from build123d import *

# Parameters (mm, degrees)
SKETCH1_W           = 35
SKETCH1_H           = 45
BOSS_EXTRUDE1_DEPTH = 6
SKETCH2_W           = 45
SKETCH2_H           = 17
BOSS_EXTRUDE2_DEPTH = 5
SKETCH3_R           = 1
CUT_EXTRUDE1_DEPTH  = 5
SKETCH3_2_R         = 1
CUT_EXTRUDE2_DEPTH  = 30
SKETCH4_R           = 2
CUT_EXTRUDE3_DEPTH  = 5
FILLET1_R           = 0.762
FILLET2_R           = 10
FILLET3_R           = 1
CUT_EXTRUDE4_DEPTH  = 23
SKETCH6_R           = 1.5
CUT_EXTRUDE5_DEPTH  = 6


with BuildPart() as part:
    # Sketch1 → Boss-Extrude1 (new body)
    with BuildSketch(Plane(origin=(0, 0, 0), x_dir=(1, 0, 0), z_dir=(0, 1, 0))):
        Rectangle(SKETCH1_W, SKETCH1_H)
    extrude(amount=BOSS_EXTRUDE1_DEPTH)

    # Sketch2 → Boss-Extrude2 (add)
    with BuildSketch(Plane.ZY.offset(17.5)):
        with Locations((0, 14.5)):
            Rectangle(SKETCH2_W, SKETCH2_H)
    boss_extrude2 = extrude(amount=-BOSS_EXTRUDE2_DEPTH)

    # Mirror1: Boss-Extrude2 across plane
    add(boss_extrude2.mirror(Plane(origin=(0, 0, 0), x_dir=(0, 0, 1), z_dir=(1, 0, 0))))

    # Sketch3 → Cut-Extrude1 (cut)
    with BuildSketch(Plane(origin=(-12.5, 0, 0), x_dir=(0, 0, -1), z_dir=(1, 0, 0))):
        with Locations((14.5, 11)):
            Circle(SKETCH3_R)
        with BuildLine():
            ThreePointArc((14.5, 17), (10.257359313, 15.242640687), (8.5, 11))
            ThreePointArc((8.5, 11), (9.5, 10), (10.5, 11))
            ThreePointArc((10.5, 11), (11.671572875, 13.828427125), (14.5, 15))
            ThreePointArc((14.5, 15), (15.5, 16), (14.5, 17))
        make_face()
    extrude(amount=-CUT_EXTRUDE1_DEPTH, mode=Mode.SUBTRACT)

    # Sketch3<2> → Cut-Extrude2 (cut)
    with BuildSketch(Plane(origin=(-12.5, 0, 0), x_dir=(0, 0, -1), z_dir=(1, 0, 0))):
        with Locations((14.5, 11)):
            Circle(SKETCH3_2_R)
    extrude(amount=CUT_EXTRUDE2_DEPTH, mode=Mode.SUBTRACT)

    # Sketch4 → Cut-Extrude3 (cut)
    with BuildSketch(Plane.ZY.offset(17.5)):
        with Locations((-14.5, 16)):
            Circle(SKETCH4_R)
    extrude(amount=-CUT_EXTRUDE3_DEPTH, mode=Mode.SUBTRACT)

    # Fillet1
    fillet1_edges = [part.edges().sort_by_distance(p)[0] for p in [
        (-12.5, 6, 0),
        (12.5, 6, 0),
    ]]
    fillet(fillet1_edges, radius=FILLET1_R)

    # Fillet2
    fillet2_edges = [part.edges().sort_by_distance(p)[0] for p in [
        (-15, 23, -22.5),
        (-15, 23, 22.5),
        (15, 23, 22.5),
        (15, 23, -22.5),
    ]]
    fillet(fillet2_edges, radius=FILLET2_R)

    # Fillet3
    fillet3_edges = [part.edges().sort_by_distance(p)[0] for p in [
        (-15, 16.7, -12.6265006),
        (-15, 14.7, -12.980131585),
    ]]
    fillet(fillet3_edges, radius=FILLET3_R)

    # Sketch5 → Cut-Extrude4 (cut)
    with BuildSketch(Plane.XZ):
        with BuildLine():
            Line((17.5, 22.5), (17.5, -5.5))
            ThreePointArc((17.5, -5.5), (0, 5.455076458), (-17.5, -5.5))
            Line((-17.5, -5.5), (-17.5, 22.5))
            Line((-17.5, 22.5), (17.5, 22.5))
        make_face()
    extrude(amount=-CUT_EXTRUDE4_DEPTH, mode=Mode.SUBTRACT)

    # Sketch6 → Cut-Extrude5 (cut)
    with BuildSketch(Plane(origin=(0, 6, 0), x_dir=(1, 0, 0), z_dir=(0, 1, 0))):
        with Locations((0, 11)):
            Circle(SKETCH6_R)
        with Locations((0, 6)):
            Circle(SKETCH6_R)
    extrude(amount=-CUT_EXTRUDE5_DEPTH, mode=Mode.SUBTRACT)


solid = part.part
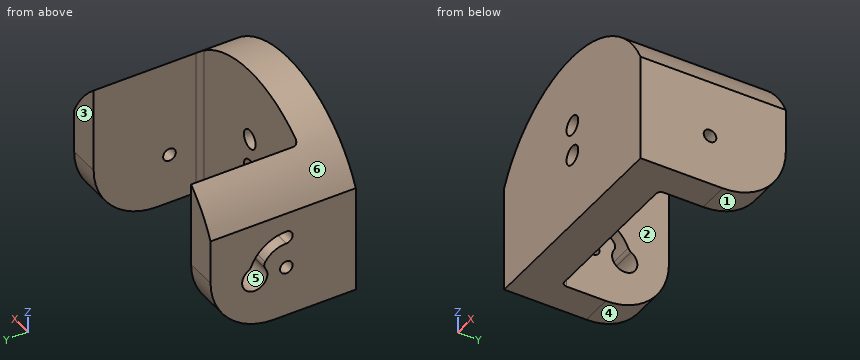
Here's how the part is built. I have some questions about the finished solid (model axes, mm). Face numbers are marked on the shaded views. A direction names the side the tool comes from. Coordinates: 2 decimals unless noted, no trailing zeros. Order: outer loops, then holes, each group sorted by start corner. A loop starts at its lowest first (then second) coordinate and runs counter-clockwise, first axis right, second up. Notation, with made-up numbers: M 86,87 L 117,87 A25 ccw 117,110 Z; hole C 66,56.5 d8. An arc over 180 degrees is marked long. Answer as CSV lines item,"result".
Item 1: We'd pull the mould along Z, two halves only. Please class the marked faces 3, 4, 5 and 6: +Z half, -Z half, draft (parallel to the pull), parting line (faces both ways), or undercut.
Results found:
face 3,"draft"
face 4,"-Z half"
face 5,"undercut"
face 6,"+Z half"
Item 2: Imagine slicing it at B-B on x = 0. Write out the boundary of the cut face in (y, z).
Results found:
outline,"M 0,-22.5 L 6,-22.5 L 6,-12.5 L 0,-12.5 Z; M 0,-9.5 L 6,-9.5 L 6,-7.5 L 0,-7.5 Z; M 0,-4.5 L 6,-4.5 L 6,5.46 L 0,5.46 Z"
Item 3: Imagine slicing it at D-D on z = -11. Write out the boundary of the cut face in (x, y), plus the area to 3 significant figures.
Results found:
outline,"M -17.5,0 L -1.5,0 L -1.5,6 L -11.74,6 A0.76 cw -12.5,6.76 L -12.5,12.94 L -17.5,12.94 Z; M -17.5,15.87 L -12.5,15.87 L -12.5,23 L -17.5,23 Z; M 1.5,0 L 17.5,0 L 17.5,23 L 12.5,23 L 12.5,6.76 A0.76 cw 11.74,6 L 1.5,6 Z"
area,"348 mm2"
Item 4: On a 3-axis mill with a long thin cutter (end or side, diameter ignored), from which of +Z, -Z, +X, -X, +Y, -Y can I reach the whole of each face in a straight line? I mean the marked faces 1 and 2. Say none if no direction works.
Results found:
face 1,"-Z, +X, -X, +Y"
face 2,"+Z, -Z, +Y"
Item 5: Imagine slicing it at C-C on y = 4. Write out the boundary of the cut face in (x, z), plus the area to 3 significant figures.
Results found:
outline,"M -17.5,-22.5 L 17.5,-22.5 L 17.5,-5.5 A19.46 ccw -17.5,-5.5 Z; hole C 0,-11 d3; hole C 0,-6 d3"
area,"856 mm2"
Item 6: Imagine slicing it at A-A on y = 7.5. Write out the boundary of the cut face in (x, z).
Results found:
outline,"M -17.5,-22.5 L -12.5,-22.5 L -12.5,0.91 A19.46 ccw -17.5,-5.5 Z; M 12.5,-22.5 L 17.5,-22.5 L 17.5,-5.5 A19.46 ccw 12.5,0.91 Z"
Item 7: For pin 1 (8 mm diameter, centred on x = -1.5, y = 11, fed in from +Z); pin 2 (2 mm diameter, centred on x = -6, z = 2, fed in from +Y), each with a flat end and sliding along its axis, tell me the tip position at first contact or that it passes through.
Results found:
pin 1,"through"
pin 2,"y = 6"
Item 8: If I drill on line 1 (X direction, y = 18.5, z = -14.5); line 2 (Y direction, x = -16.15, z = -14.5); line 3 (Z direction, x = 0, y = 4), over which ranges is the centre line in solid material (lowest first)?
Results found:
line 1,"-17.5 to -12.5, 12.5 to 17.5"
line 2,"0 to 10, 12 to 14, 18 to 22.8"
line 3,"-22.5 to -12.5, -9.5 to -7.5, -4.5 to 5.46"
